```python
from build123d import *

# Parameters (mm, degrees)
SKETCH1_R                = 25
BOSS_EXTRUDE1_DEPTH      = 200
SKETCH2_R                = 25
BOSS_EXTRUDE2_DEPTH      = 20
BOSS_EXTRUDE2_DEPTH_BACK = 220
CUT_EXTRUDE1_START       = -50
SKETCH3_W                = 128.293241695
SKETCH3_H                = 120
CUT_EXTRUDE1_DEPTH       = 100


with BuildPart() as part:
    # Sketch1 → Boss-Extrude1 (new body)
    with BuildSketch(Plane.XY):
        with BuildLine():
            Line((28.722813233, -20), (396.277186767, -20))
            ThreePointArc((396.277186767, -20), (456.024184115, -16.201851746), (425, 35))
            Line((425, 35), (425, 80))
            Line((425, 80), (0, 80))
            Line((0, 80), (0, 35))
            ThreePointArc((0, 35), (-31.024184115, -16.201851746), (28.722813233, -20))
        make_face()
        with Locations((425, 0)):
            Circle(SKETCH1_R, mode=Mode.SUBTRACT)
    extrude(amount=BOSS_EXTRUDE1_DEPTH)

    # Sketch2 → Boss-Extrude2 (add, two sides)
    with BuildSketch(Plane.XY.offset(200)) as boss_extrude2_sk:
        Circle(SKETCH2_R)
    extrude(amount=BOSS_EXTRUDE2_DEPTH)
    extrude(boss_extrude2_sk.sketch, amount=-BOSS_EXTRUDE2_DEPTH_BACK)

    # Sketch3 → Cut-Extrude1 (cut)
    with BuildSketch(Plane.XY.offset(200).offset(CUT_EXTRUDE1_START)):
        with Locations((429.146620848, 20)):
            Rectangle(SKETCH3_W, SKETCH3_H)
    extrude(amount=-CUT_EXTRUDE1_DEPTH, mode=Mode.SUBTRACT)


solid = part.part
```
The listing builds one solid part. Answer for the finished solid, in the listing's coordinates (mm). A direction names the side the tool comes from. Coordinates: 2 decimals unless noted, no trailing zeros. Order: outer loops, then holes, each group sorted by start corner. A loop starts at its lowest first (then second) coordinate and runs counter-clockwise, first axis right, second up. Notation, with made-up numbers: M 6,79.25 L 25,79.25 A19 cw 25,103.25 Z; hole C 21,10 d1. An arc over 180 degrees is marked long. Answer as a JSON object with one key per item and string values. Group by question number.
1. Flat-ended cylindrical pins translate along their axes: P1, Ø1, axis at x = 118, z = 83, coming from the -Y side; P2, Ø3, axis at x = 390, y = 40, coming from the -Z side; P3, Ø2, axis at y = -16, z = 6.5, coming from the +X side. Find the tip coordinate at first contact, or state that the pin passes through.
2. Section B-B on z = 30.5 is taken. Write down the section's boundary in (x, y).
3. Section D-D on z = 123.5 is taken. Write down the section's boundary in (x, y), then the cut area to 3 significant figures.
4. Section C-C on y = 59.5 is taken. Write down the section's boundary in (x, z), then the cut area to 3 significant figures.
5. Determine the mould class of faces 1 (the flat face through (0, 0, -20)), 2 (the flat face through (425, 57, 25)), 3 (the flat face through (210, -20, 99)) for opening direction X: released by +X, released by -X, zero draft, split by the parting line, or undercut.
6. Section A-A on y = 0 is taken. Write down the section's boundary in (x, z), then the cut area to 3 significant figures.
7. Straight lines are drawn through the part: line 1 (X direction, y = 0, z = 22); line 2 (X direction, y = -21.5, z = 8); line 3 (X direction, y = 44.5, z = 144). For each, find the intervals that lie inside material, in ascending order.
8. A tool of negligible diameter and unlimited length cuts with its end or side. For faces 4 (the cylindrical face through (23.846, 7.509, 209.86)), 5 (the flat face through (425, 57, 175)), 6 (the flat face through (0, 58, 99)), 7 (the flat face through (401, 23, 150)), 8 (the cylindrical face through (23.846, 7.509, -9.86)), from which of +Z, -Z, +X, -X, +Y, -Y can it reach the whole face along a straight path? Write none if from no direction.
Values follow:
{
 "1": {"P1": "y = -20", "P2": "z = 0", "P3": "x = 456.62"},
 "2": {"outline": "M 0,35 A35 ccw long 28.72,-20 L 396.28,-20 A35 ccw long 425,35 L 425,80 L 0,80 Z; hole C 425,0 d50"},
 "3": {"outline": "M 0,35 A35 ccw long 28.72,-20 L 365,-20 L 365,80 L 0,80 Z", "area": "38,700 mm2"},
 "4": {"outline": "M 0,0 L 425,0 L 425,50 L 365,50 L 365,150 L 425,150 L 425,200 L 0,200 Z", "area": "79,000 mm2"},
 "5": {"face 1": "zero draft", "face 2": "released by +X", "face 3": "undercut"},
 "6": {"outline": "M -35,0 L -25,0 L -25,-20 L 25,-20 L 25,0 L 400,0 L 400,50 L 365,50 L 365,150 L 400,150 L 400,200 L 25,200 L 25,220 L -25,220 L -25,200 L -35,200 Z; M 450,0 L 460,0 L 460,50 L 450,50 Z; M 450,150 L 460,150 L 460,200 L 450,200 Z", "area": "86,500 mm2"},
 "7": {"line 1": "-35 to 400, 450 to 460", "line 2": "-27.62 to 27.62, 397.38 to 412.24, 437.76 to 452.62", "line 3": "0 to 365"},
 "8": {"face 4": "+Z", "face 5": "+Z, -Z, +X, +Y", "face 6": "+Z, -Z, -X, +Y", "face 7": "+X, +Y, -Y", "face 8": "-Z"}
}
